Verification items for this drawing (mm, ordinates from the low corner). Give positions to 0.01 mm unless a question says otherwise; leave off trailing zeros. Order: outer loops, then holes, each group sorted by start corner. A loop starts at its lowest first (then second) coordinate and runs counter-clockwise, first axis right, second up. Notation, with made-up numbers: (-3, 27.5) - (12, 27.5) arc R14 cw to (12, 36.5) - close; hole circle Ø7 at (-25.75, 25.25). An arc over 180 degrees is marked (long way). Put each result on its own line as item: value. Start each with the question number.
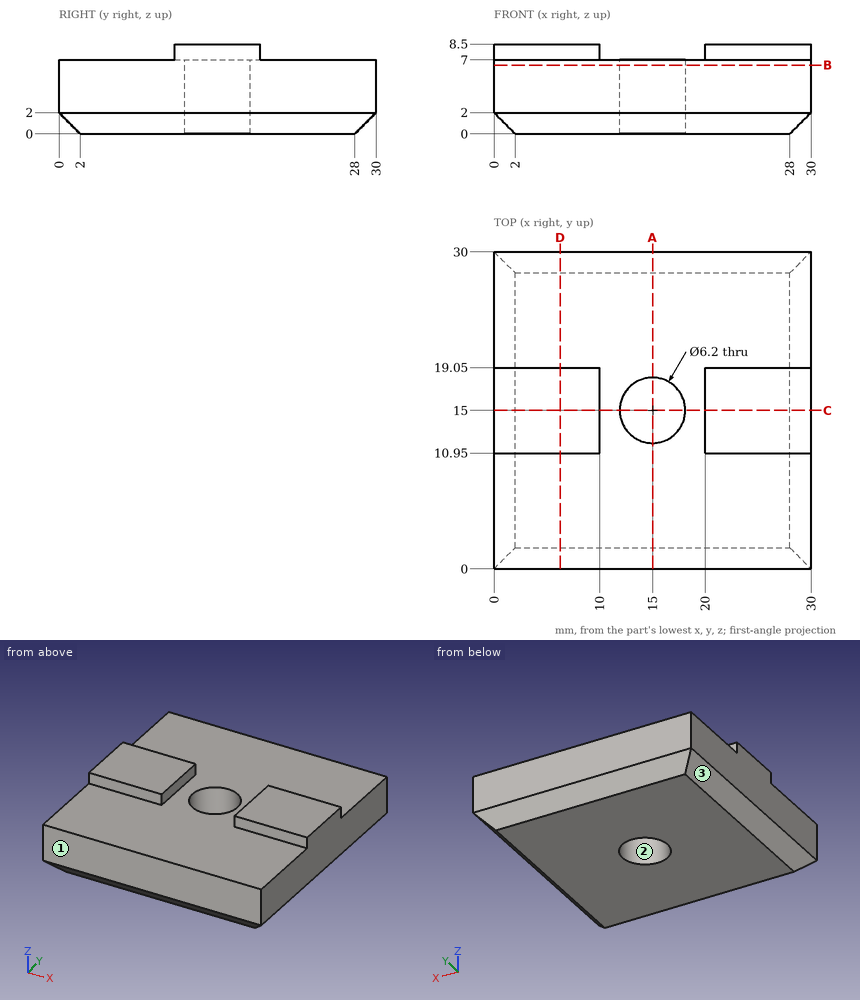
Item 1: Gauge pin test, flat ends, axial feed: pin 1 Ø15 at (x, y) = (12, 16.5) entering from +Z; pin 2 Ø1.5 at (x, y) = (8, 3.5) entering from +Z; pin 3 Ø1.2 at (x, z) = (25, 8) entering from +Y. Record the tip position at first contact, or that the pin passes through.
Item 2: Release check for a two-part mould opening along Y. For the marked faces 1, 2 and 3 record: +Y half, -Y half, draft (parallel to the pull), parting line (faces both ways), or undercut.
Item 3: Thickness scan on line 1 along Y through (x, z) = (15, 4); line 2 along Z through (x, y) = (18.25, 14.75); line 3 along Y through (x, z) = (2, 8). Record the ranges inside material, lowest first.
Item 4: Cross-section at C-C (y = 15). Enter the section's corners in (x, z).
Item 5: Cross-section at D-D (x = 6.25). Enter the section's corners in (y, z), and give its area (3 significant figures).
Item 6: Cross-section at B-B (z = 6.5). Enter the section's corners in (x, y).
Item 7: Cross-section at A-A (x = 15). Enter the section's corners in (y, z), and give its area (3 significant figures).
Recorded:
1. pin 1: stops at z = 8.5
1. pin 2: stops at z = 7
1. pin 3: stops at y = 19.05
2. face 1: -Y half
2. face 2: undercut
2. face 3: draft
3. line 1: y = 0 to 11.9, 18.1 to 30
3. line 2: z = 0 to 7
3. line 3: y = 10.95 to 19.05
4. outline: (0, 2) - (2, 0) - (11.9, 0) - (11.9, 7) - (10, 7) - (10, 8.5) - (0, 8.5) - close; (18.1, 0) - (28, 0) - (30, 2) - (30, 8.5) - (20, 8.5) - (20, 7) - (18.1, 7) - close
5. outline: (0, 2) - (2, 0) - (28, 0) - (30, 2) - (30, 7) - (19.05, 7) - (19.05, 8.5) - (10.95, 8.5) - (10.95, 7) - (0, 7) - close
5. area: 218 mm^2
6. outline: (0, 0) - (30, 0) - (30, 30) - (0, 30) - close; hole circle Ø6.2 at (15, 15)
7. outline: (0, 2) - (2, 0) - (11.9, 0) - (11.9, 7) - (0, 7) - close; (18.1, 0) - (28, 0) - (30, 2) - (30, 7) - (18.1, 7) - close
7. area: 163 mm^2
